```python
from build123d import *

# Parameters (mm, degrees)
SKETCH1_W           = 38.1
SKETCH1_H           = 14
BOSS_EXTRUDE1_DEPTH = 7
FILLET1_R           = 2.54
CUT_EXTRUDE1_DEPTH  = 12.7
FILLET2_R           = 1
FILLET3_R           = 0.25


with BuildPart() as part:
    # Sketch1 → Boss-Extrude1 (new, symmetric)
    with BuildSketch(Plane.XY):
        with Locations((19.05, 7)):
            Rectangle(SKETCH1_W, SKETCH1_H)
    extrude(amount=BOSS_EXTRUDE1_DEPTH, both=True)

    # Fillet1
    fillet1_edges = [part.edges().sort_by_distance(p)[0] for p in [
        (38.1, 7, 7),
        (19.05, 14, 7),
        (0, 7, 7),
        (19.05, 14, -7),
        (38.1, 7, -7),
        (19.05, 0, -7),
        (0, 7, -7),
        (19.05, 0, 7),
        (0, 14, 0),
        (38.1, 14, 0),
        (38.1, 0, 0),
        (0, 0, 0),
    ]]
    fillet(fillet1_edges, radius=FILLET1_R)

    # Sketch3 → Cut-Extrude1 (cut)
    with BuildSketch(Plane(origin=(-2.317550632, 13.143482763, 0), x_dir=(0.9848077530122074, 0.1736481776669347, 0), z_dir=(-0.17364817766693472, 0.9848077530122075, 0))):
        Polygon((16.548510348, 0), (14.527784405, 3.5), (10.486332521, 3.5), (8.465606579, 0), (10.486332521, -3.5), (14.527784405, -3.5), align=None)
    extrude(amount=-CUT_EXTRUDE1_DEPTH, mode=Mode.SUBTRACT)

    # Fillet2
    fillet2_edges = [part.edges().sort_by_distance(p)[0] for p in [
        (15.189869229, 3.334595276, 1.75),
        (12.204829367, 2.80825221, 3.5),
        (9.219789505, 2.281909144, 1.75),
        (9.219789505, 2.281909144, -1.75),
        (12.204829367, 2.80825221, -3.5),
        (15.189869229, 3.334595276, -1.75),
    ]]
    fillet(fillet2_edges, radius=FILLET2_R)

    # Fillet3
    fillet3_edges = [part.edges().sort_by_distance(p)[0] for p in [
        (13.152264465, 9.07197767, 3.5),
        (9.110338994, 8.721082293, 3.5),
        (7.089376258, 8.545634604, 0),
        (9.110338994, 8.721082293, -3.5),
        (13.152264465, 9.07197767, -3.5),
        (15.173227201, 9.247425359, 0),
        (10.349377707, 2.753337988, -3.181429078),
        (13.96716537, 3.391251564, -3.181429078),
        (8.540483876, 2.434381201, 0),
        (15.776059261, 3.71020842, 0),
        (10.349377707, 2.753337988, 3.181429078),
        (13.96716537, 3.391251564, 3.181429078),
    ]]
    fillet(fillet3_edges, radius=FILLET3_R)


solid = part.part
```
Work out the finished part from the listing and answer in its coordinate system (mm). A direction names the side the tool comes from. Coordinates: 2 decimals unless noted, no trailing zeros. Write each loop counter-clockwise with the first axis right and the second up, starting at its lowest first coordinate (ties: lowest second). Pieces come first, ordered by that corner, then holes.
Q1. Which of the six approach directions +Z, -Z, +X, -X, +Y, -Y give full straight-line access (tool end or side, diameter ignored) to faces 1 (the face through (12.2, 3.1, 3.2)), 2 (the face through (8.06, 8.79, 1.73)), 3 (the face through (38.1, 7, 0))?
Q2. A cutting plane is placed at A-A, the plane x = 22. Give the vertices of the cut face in (y, z), then the cut area to 3 significant figures.
Q3. Find the intervals of material crossed by line 1 (Z direction, x = 12.5, y = 4.5); line 2 (Z direction, x = 7, y = 12.75); line 3 (X direction, y = 6.25, z = -3.25), in increasing order.
Q4. A cutting plane is placed at B-B, the plane z = 5. Give the vertices of the cut face in (x, y).
Q5. This flat-tipped pin is pushed along its axis until it touches: pin 1 Ø3 at (x, z) = (10.5, -5.5) entering from -Y. Where does it stop, or does it pass through?
Q6. Determine the mould class of faces 4 (the face through (19, 0, 0)), 5 (the face through (19.281, 0.764, -6.276)), 6 (the face through (9.424, 2.623, 1.63)) for opening direction Z: released by +Z, released by -Z, zero draft, split by the parting line, or undercut.
Findings below:
1. face 1: none
1. face 2: +Y
1. face 3: +Z, -Z, +X, +Y, -Y
2. outline: (0, -4.46) arc R2.54 ccw to (2.54, -7) - (11.46, -7) arc R2.54 ccw to (14, -4.46) - (14, 4.46) arc R2.54 ccw to (11.46, 7) - (2.54, 7) arc R2.54 ccw to (0, 4.46) - close
2. area: 190 mm2
3. line 1: z = -7 to -3.5, 3.5 to 7
3. line 2: z = -6.65 to -1.11, 1.11 to 6.65
3. line 3: x = 0 to 9.4, 13.8 to 38.1
4. outline: (0.06, 2.54) arc R2.48 ccw to (2.54, 0.06) - (35.56, 0.06) arc R2.48 ccw to (38.04, 2.54) - (38.04, 11.46) arc R2.48 ccw to (35.56, 13.94) - (2.54, 13.94) arc R2.48 ccw to (0.06, 11.46) - close
5. pin 1: stops at y = 0
6. face 4: zero draft
6. face 5: released by -Z
6. face 6: undercut
